Input: part model. Units: mm. Frame: model coordinates. Face numbers are marked on the shaded views. A direction names the side the tool comes from. Give positions to 0.01 mm unless a question says otherwise; leave off trailing zeros. Write each loop counter-clockwise with the first axis right and the second up, starting at its lowest first coordinate (ties: lowest second). Pieces come first, ordered by that corner, then holes.
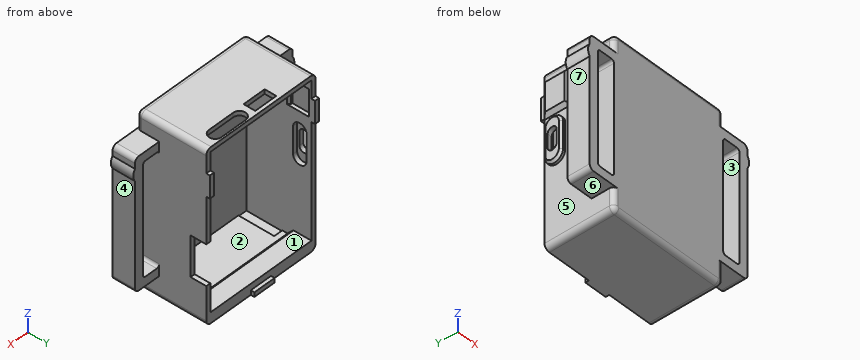
```python
from build123d import *

# Parameters (mm, degrees)
SKETCH_1_W          = 27
SKETCH_1_H          = 38
EXTRUDE_1_DEPTH     = 1
SKETCH_3_W          = 27
SKETCH_3_H          = 38
SKETCH_3_W_2        = 25
SKETCH_3_H_2        = 36
EXTRUDE_2_DEPTH     = 14.5
FILLET_1_R          = 1.2
EXTRUDE_3_DEPTH     = 5
FILLET_3_R          = 1
FILLET_4_R          = 0.6
FILLET_6_R          = 1
CUT_EXTRUDE_1_REACH = 47.437
CUT_EXTRUDE_2_REACH = 43.113
SKETCH_6_W          = 9
SKETCH_6_H          = 3.5
EXTRUDE_4_DEPTH     = 5
CUT_EXTRUDE_3_REACH = 47.61
SKETCH_8_W          = 5.2
SKETCH_8_H          = 2.6
SKETCH_13_W         = 6
SKETCH_13_H         = 4
CUT_EXTRUDE_6_DEPTH = 0.8
SKETCH_15_W         = 25
SKETCH_15_H         = 5
EXTRUDE_5_DEPTH     = 1.4
CHAMFER_3_SIZE      = 1
SKETCH_16_W         = 2
SKETCH_16_H         = 0.2
CUT_EXTRUDE_7_DEPTH = 8
SKETCH_18_W         = 5
SKETCH_18_H         = 1
SKETCH_18_W_2       = 1
SKETCH_18_H_2       = 5
EXTRUDE_6_DEPTH     = 0.8
EXTRUDE_9_DEPTH     = 1
CUT_EXTRUDE_8_REACH = 44.545
CUT_EXTRUDE_9_DEPTH = 1
CHAMFER_4_SIZE      = 0.5
SKETCH_22_W         = 8
SKETCH_22_H         = 6
EXTRUDE_10_DEPTH    = 0.8
CHAMFER_6_SIZE      = 0.8
CHAMFER_7_SIZE      = 0.5


with BuildPart() as part:
    # 草图1 → 凸台-拉伸1 (new body)
    with BuildSketch(Plane(origin=(0, 0, 0), x_dir=(1, 0, 0), z_dir=(0, 1, 0))):
        Rectangle(SKETCH_1_W, SKETCH_1_H)
    extrude(amount=EXTRUDE_1_DEPTH)

    # 草图3 → 凸台-拉伸2 (add)
    with BuildSketch(Plane(origin=(0, 1, 0), x_dir=(1, 0, 0), z_dir=(0, 1, 0))):
        Rectangle(SKETCH_3_W, SKETCH_3_H)
        Rectangle(SKETCH_3_W_2, SKETCH_3_H_2, mode=Mode.SUBTRACT)
    extrude(amount=EXTRUDE_2_DEPTH)

    # 圆角1
    fillet_1_edges = [part.edges().sort_by_distance(p)[0] for p in [
        (13.5, 7.75, 19),
        (-13.5, 7.75, 19),
        (-13.5, 7.75, -19),
        (13.5, 7.75, -19),
    ]]
    fillet(fillet_1_edges, radius=FILLET_1_R)

    # 草图4 → 凸台-拉伸3 (add)
    with BuildSketch(Plane.XZ):
        Polygon((13.5, 15), (19.5, 15), (19.5, -14), (13.5, -14), (13.5, -12), (17.5, -12), (17.5, 13), (13.5, 13), align=None)
        Polygon((-17.5, 13), (-17.5, -12), (-13.5, -12), (-13.5, -14), (-19.5, -14), (-19.5, 15), (-13.5, 15), (-13.5, 13), align=None)
    extrude(amount=-EXTRUDE_3_DEPTH)

    # 圆角3
    fillet_3_edges = [part.edges().sort_by_distance(p)[0] for p in [
        (19.5, 2.5, 15),
        (19.5, 2.5, -14),
        (-19.5, 2.5, -14),
        (-19.5, 2.5, 15),
    ]]
    fillet(fillet_3_edges, radius=FILLET_3_R)

    # 圆角4
    fillet_4_edges = [part.edges().sort_by_distance(p)[0] for p in [
        (13.5, 2.5, 13),
        (13.5, 2.5, -12),
        (17.5, 2.5, -12),
        (17.5, 2.5, 13),
        (-13.5, 2.5, 13),
        (-17.5, 2.5, 13),
        (-17.5, 2.5, -12),
        (-13.5, 2.5, -12),
    ]]
    fillet(fillet_4_edges, radius=FILLET_4_R)

    # 圆角6
    fillet_6_edges = [part.edges().sort_by_distance(p)[0] for p in [
        (0, 0, -19),
        (13.5, 0, 16.4),
        (0, 0, 19),
        (-13.5, 0, -15.9),
        (13.148528137, 0, 18.648528137),
        (-13.148528137, 0, 18.648528137),
        (-13.148528137, 0, -18.648528137),
        (13.148528137, 0, -18.648528137),
        (13.5, 0, -15.9),
        (-13.5, 0, 16.4),
    ]]
    fillet(fillet_6_edges, radius=FILLET_6_R)

    # 草图5 → 切除-拉伸1 (cut, up to next)
    with BuildSketch(Plane.XY.offset(19), mode=Mode.PRIVATE) as cut_extrude_1_sk1:
        with BuildLine():
            Line((3.3, 15.1), (9.3, 15.1))
            ThreePointArc((9.3, 15.1), (10.7, 13.7), (9.3, 12.3))
            Line((9.3, 12.3), (3.3, 12.3))
            ThreePointArc((3.3, 12.3), (1.9, 13.7), (3.3, 15.1))
        make_face()
    cut_extrude_1_tool1 = extrude(cut_extrude_1_sk1.sketch, amount=-CUT_EXTRUDE_1_REACH, mode=Mode.PRIVATE) & part.part
    add(cut_extrude_1_tool1.solids().sort_by_distance((6.3, 13.7, 19))[0], mode=Mode.SUBTRACT)

    # 草图6 → 切除-拉伸2 (cut, up to next)
    with BuildSketch(Plane(origin=(13.5, 0, 0), x_dir=(0, 0, -1), z_dir=(1, 0, 0)), mode=Mode.PRIVATE) as cut_extrude_2_sk1:
        with Locations((5.8, 13.75)):
            Rectangle(SKETCH_6_W, SKETCH_6_H)
    cut_extrude_2_tool1 = extrude(cut_extrude_2_sk1.sketch, amount=-CUT_EXTRUDE_2_REACH, mode=Mode.PRIVATE) & part.part
    add(cut_extrude_2_tool1.solids().sort_by_distance((13.5, 13.75, -5.8))[0], mode=Mode.SUBTRACT)

    # 草图7 → 凸台-拉伸4 (add)
    with BuildSketch(Plane.XZ):
        with BuildLine():
            Line((19.5, 12.826649916), (19.5, 10.173350084))
            ThreePointArc((19.5, 10.173350084), (19.9, 11.5), (19.5, 12.826649916))
        make_face()
        with BuildLine():
            Line((-19.5, 12.826649916), (-19.5, 10.173350084))
            ThreePointArc((-19.5, 10.173350084), (-19.9, 11.5), (-19.5, 12.826649916))
        make_face()
    extrude(amount=-EXTRUDE_4_DEPTH)

    # 草图8 → 切除-拉伸3 (cut, up to next)
    with BuildSketch(Plane.XY.offset(19), mode=Mode.PRIVATE) as cut_extrude_3_sk1:
        with Locations((-2.1, 13.4)):
            Rectangle(SKETCH_8_W, SKETCH_8_H)
    cut_extrude_3_tool1 = extrude(cut_extrude_3_sk1.sketch, amount=-CUT_EXTRUDE_3_REACH, mode=Mode.PRIVATE) & part.part
    add(cut_extrude_3_tool1.solids().sort_by_distance((-2.1, 13.4, 19))[0], mode=Mode.SUBTRACT)

    # 草图13 → 切除-拉伸6 (cut)
    with BuildSketch(Plane(origin=(-12.5, 0, 0), x_dir=(0, 0, -1), z_dir=(1, 0, 0))):
        with Locations((-12.8, 12.5)):
            Rectangle(SKETCH_13_W, SKETCH_13_H)
    extrude(amount=-CUT_EXTRUDE_6_DEPTH, mode=Mode.SUBTRACT)

    # 草图15 → 凸台-拉伸5 (add)
    with BuildSketch(Plane.XY.offset(-18)):
        with Locations((0, 13)):
            Rectangle(SKETCH_15_W, SKETCH_15_H)
    extrude(amount=EXTRUDE_5_DEPTH)

    # 倒角3
    chamfer_3_edges = [part.edges().sort_by_distance(p)[0] for p in [
        (0, 10.5, -16.6),
    ]]
    chamfer(chamfer_3_edges, length=CHAMFER_3_SIZE)

    # 草图16 → 切除-拉伸7 (cut)
    with BuildSketch(Plane(origin=(0, 1, 0), x_dir=(1, 0, 0), z_dir=(0, 1, 0))):
        with Locations((-11.5, 18.1)):
            Rectangle(SKETCH_16_W, SKETCH_16_H)
        with Locations((11.1, 18.1)):
            Rectangle(SKETCH_16_W, SKETCH_16_H)
    extrude(amount=CUT_EXTRUDE_7_DEPTH, mode=Mode.SUBTRACT)

    # 草图18 → 凸台-拉伸6 (add)
    with BuildSketch(Plane(origin=(0, 15.5, 0), x_dir=(1, 0, 0), z_dir=(0, 1, 0))):
        with Locations((0, 18.5)):
            Rectangle(SKETCH_18_W, SKETCH_18_H)
        with Locations((-13, -11.5)):
            Rectangle(SKETCH_18_W_2, SKETCH_18_H_2)
        with Locations((13, -11.5)):
            Rectangle(SKETCH_18_W_2, SKETCH_18_H_2)
    extrude(amount=EXTRUDE_6_DEPTH)

    # 草图19 → 凸台-拉伸9 (add)
    with BuildSketch(Plane.ZY.offset(13.5)):
        with BuildLine():
            Line((-0.2, 14.9), (5.8, 14.9))
            ThreePointArc((5.8, 14.9), (7.8, 12.9), (5.8, 10.9))
            Line((5.8, 10.9), (-0.2, 10.9))
            ThreePointArc((-0.2, 10.9), (-2.2, 12.9), (-0.2, 14.9))
        make_face()
    extrude(amount=EXTRUDE_9_DEPTH)

    # 草图20 → 切除-拉伸8 (cut, up to next)
    with BuildSketch(Plane.ZY.offset(14.5), mode=Mode.PRIVATE) as cut_extrude_8_sk1:
        with BuildLine():
            Line((1.3, 13.9), (4.3, 13.9))
            ThreePointArc((4.3, 13.9), (5.3, 12.9), (4.3, 11.9))
            Line((4.3, 11.9), (1.3, 11.9))
            ThreePointArc((1.3, 11.9), (0.3, 12.9), (1.3, 13.9))
        make_face()
    cut_extrude_8_tool1 = extrude(cut_extrude_8_sk1.sketch, amount=-CUT_EXTRUDE_8_REACH, mode=Mode.PRIVATE) & part.part
    add(cut_extrude_8_tool1.solids().sort_by_distance((-14.5, 12.9, 2.8))[0], mode=Mode.SUBTRACT)

    # 草图21 → 切除-拉伸9 (cut)
    with BuildSketch(Plane(origin=(-12.5, 0, 0), x_dir=(0, 0, -1), z_dir=(1, 0, 0))):
        with BuildLine():
            Line((-5.8, 14.4), (0.2, 14.4))
            ThreePointArc((0.2, 14.4), (1.7, 12.9), (0.2, 11.4))
            Line((0.2, 11.4), (-5.8, 11.4))
            ThreePointArc((-5.8, 11.4), (-7.3, 12.9), (-5.8, 14.4))
        make_face()
    extrude(amount=-CUT_EXTRUDE_9_DEPTH, mode=Mode.SUBTRACT)

    # 倒角4
    chamfer_4_edges = [part.edges().sort_by_distance(p)[0] for p in [
        (-14.5, 12.9, -2.2),
        (-14.5, 10.9, 2.8),
        (-14.5, 12.9, 7.8),
        (-14.5, 14.9, 2.8),
    ]]
    chamfer(chamfer_4_edges, length=CHAMFER_4_SIZE)

    # 草图22 → 凸台-拉伸10 (add)
    with BuildSketch(Plane.ZY.offset(13.5)):
        with Locations((12.8, 12.5)):
            Rectangle(SKETCH_22_W, SKETCH_22_H)
    extrude(amount=EXTRUDE_10_DEPTH)

    # 倒角6
    chamfer_6_edges = [part.edges().sort_by_distance(p)[0] for p in [
        (-14.3, 12.5, 16.8),
        (-14.3, 9.5, 12.8),
        (-14.3, 15.5, 12.8),
        (-14.3, 12.5, 8.8),
    ]]
    chamfer(chamfer_6_edges, length=CHAMFER_6_SIZE - 0.0001)  # a hair under: the kernel refuses the full size

    # 倒角7
    chamfer_7_edges = [part.edges().sort_by_distance(p)[0] for p in [
        (-12.5, 10.5, 12.8),
        (-12.5, 14.5, 12.8),
    ]]
    chamfer(chamfer_7_edges, length=CHAMFER_7_SIZE)


solid = part.part
```
Q1. Pin query (flat end, axial travel): pin 1 (1.1 mm diameter, centred on x = 13, z = 3, fed in from +Y); pin 2 (8 mm diameter, centred on x = 1.5, z = -9, fed in from +Y); pin 3 (1.5 mm diameter, centred on y = 14, z = -9.5, fed in from +X). Return the tip coordinate at first contact, or that it passes through.
Q2. Material intervals for line 1 along Z through (x, y) = (8.5, 5.75); line 2 along X through (y, z) = (5.25, -6.5); line 3 along X through (y, z) = (3, -4.5), sorted ascending.
Q3. Section A-A, the plane x = -15. Return the cut outline in (y, z), then the cut area to 3 significant figures.
Q4. Section C-C, the plane y = 6.25. Return the cut outline in (x, z), then the cut area to 3 significant figures.
Q5. Section B-B, the plane z = -5.5. Return the cut outline in (x, y).
Q6. Section D-D, the plane x = 11.5. Return the cut outline in (y, z), then the cut area to 3 significant figures.
Q7. Mould query, pull axis Z, two halves, no side actions, for the marked faces 5, 6 and 7. Classes: +Z half, -Z half, draft (parallel to the pull), parting line (faces both ways), or undercut.
Q8. Access query for the marked faces 1, 2, 3 and 4. Directions: +Z, -Z, +X, -X, +Y, -Y. A direction counts if a zero-diameter tool reaches every point of the face in a straight line with its end or side. Return the directions, or none.
Solutions:
1. pin 1: stops at y = 15.5
1. pin 2: stops at y = 1
1. pin 3: stops at x = -12.5
2. line 1: z = -19 to -18, 18 to 19
2. line 2: x = -13.5 to -12.5, 12.5 to 13.5
2. line 3: x = -19.5 to -17.5, -13.5 to -12.5, 12.5 to 13.5, 17.5 to 19.5
3. outline: (0, -14) - (5, -14) - (5, -12) - (0, -12) - close; (0, 13) - (5, 13) - (5, 15) - (0, 15) - close
3. area: 20.0 mm2
4. outline: (-13.5, -17.8) arc R1.2 ccw to (-12.3, -19) - (12.3, -19) arc R1.2 ccw to (13.5, -17.8) - (13.5, 17.8) arc R1.2 ccw to (12.3, 19) - (-12.3, 19) arc R1.2 ccw to (-13.5, 17.8) - close; hole (-12.5, -18.2) - (-10.5, -18.2) - (-10.5, -18) - (10.1, -18) - (10.1, -18.2) - (12.1, -18.2) - (12.1, -18) - (12.5, -18) - (12.5, 18) - (-12.5, 18) - close
4. area: 124 mm2
5. outline: (-19.5, 0) - (-17.5, 0) - (-17.5, 5) - (-19.5, 5) - close; (-13.5, 0) - (13.5, 0) - (13.5, 12) - (12.5, 12) - (12.5, 1) - (-12.5, 1) - (-12.5, 15.5) - (-13.5, 15.5) - close; (17.5, 0) - (19.5, 0) - (19.5, 5) - (17.5, 5) - close
6. outline: (0, -18) arc R1 ccw to (1, -19) - (15.5, -19) - (15.5, -16.6) - (11.5, -16.6) - (10.5, -17.6) - (10.5, -18) - (9, -18) - (9, -18.2) - (1, -18.2) - (1, 18) - (15.5, 18) - (15.5, 19) - (1, 19) arc R1 ccw to (0, 18) - close
6. area: 71.5 mm2
7. face 5: undercut
7. face 6: -Z half
7. face 7: draft
8. face 1: +Y
8. face 2: none
8. face 3: +Y, -Y
8. face 4: -Z, +X, +Y, -Y
